```python
from build123d import *

# Parameters (mm, degrees)
F0_W     = 457.2
F0_H     = 304.8
F0_R     = 6.35
F1_DEPTH = 6.35
F2_W     = 2.54
F2_H     = 5.08
F3_DEPTH = 2.54


with BuildPart() as f1:
    # F0 (on Top) → F1 (new body)
    with BuildSketch(Plane.XY):
        with Locations((228.6, -152.4)):
            Rectangle(F0_W, F0_H)
        with Locations((25.4, -272.70785)):
            Circle(F0_R, mode=Mode.SUBTRACT)
        with Locations((76.2, -272.70785)):
            Circle(F0_R, mode=Mode.SUBTRACT)
        with Locations((127, -272.70785)):
            Circle(F0_R, mode=Mode.SUBTRACT)
        with Locations((177.8, -272.70785)):
            Circle(F0_R, mode=Mode.SUBTRACT)
        with Locations((25.4, -221.90785)):
            Circle(F0_R, mode=Mode.SUBTRACT)
        with Locations((76.2, -221.90785)):
            Circle(F0_R, mode=Mode.SUBTRACT)
        with Locations((25.4, -171.10785)):
            Circle(F0_R, mode=Mode.SUBTRACT)
        with Locations((76.2, -171.10785)):
            Circle(F0_R, mode=Mode.SUBTRACT)
        with Locations((127, -221.90785)):
            Circle(F0_R, mode=Mode.SUBTRACT)
        with Locations((177.8, -221.90785)):
            Circle(F0_R, mode=Mode.SUBTRACT)
        with Locations((127, -171.10785)):
            Circle(F0_R, mode=Mode.SUBTRACT)
        with Locations((177.8, -171.10785)):
            Circle(F0_R, mode=Mode.SUBTRACT)
        with Locations((228.6, -272.70785)):
            Circle(F0_R, mode=Mode.SUBTRACT)
        with Locations((279.4, -272.70785)):
            Circle(F0_R, mode=Mode.SUBTRACT)
        with Locations((330.2, -272.70785)):
            Circle(F0_R, mode=Mode.SUBTRACT)
        with Locations((381, -272.70785)):
            Circle(F0_R, mode=Mode.SUBTRACT)
        with BuildLine():
            ThreePointArc((438.15, -272.70785), (427.309872, -277.197978), (431.8, -266.35785))
            Line((431.8, -266.35785), (431.8, -262.54785))
            Line((431.8, -262.54785), (444.5, -262.54785))
            Line((444.5, -262.54785), (444.5, -272.70785))
            Line((444.5, -272.70785), (438.15, -272.70785))
        make_face(mode=Mode.SUBTRACT)
        with Locations((228.6, -221.90785)):
            Circle(F0_R, mode=Mode.SUBTRACT)
        with Locations((279.4, -221.90785)):
            Circle(F0_R, mode=Mode.SUBTRACT)
        with Locations((330.2, -221.90785)):
            Circle(F0_R, mode=Mode.SUBTRACT)
        with Locations((228.6, -171.10785)):
            Circle(F0_R, mode=Mode.SUBTRACT)
        with Locations((279.4, -171.10785)):
            Circle(F0_R, mode=Mode.SUBTRACT)
        with Locations((330.2, -171.10785)):
            Circle(F0_R, mode=Mode.SUBTRACT)
        with Locations((381, -221.90785)):
            Circle(F0_R, mode=Mode.SUBTRACT)
        with Locations((431.8, -221.90785)):
            Circle(F0_R, mode=Mode.SUBTRACT)
        with Locations((381, -171.10785)):
            Circle(F0_R, mode=Mode.SUBTRACT)
        with Locations((431.8, -171.10785)):
            Circle(F0_R, mode=Mode.SUBTRACT)
        with Locations((25.4, -120.30785)):
            Circle(F0_R, mode=Mode.SUBTRACT)
        with Locations((76.2, -120.30785)):
            Circle(F0_R, mode=Mode.SUBTRACT)
        with Locations((127, -120.30785)):
            Circle(F0_R, mode=Mode.SUBTRACT)
        with Locations((177.8, -120.30785)):
            Circle(F0_R, mode=Mode.SUBTRACT)
        with Locations((25.4, -69.50785)):
            Circle(F0_R, mode=Mode.SUBTRACT)
        with Locations((76.2, -69.50785)):
            Circle(F0_R, mode=Mode.SUBTRACT)
        with Locations((25.4, -18.70785)):
            Circle(F0_R, mode=Mode.SUBTRACT)
        with Locations((76.2, -18.70785)):
            Circle(F0_R, mode=Mode.SUBTRACT)
        with Locations((127, -69.50785)):
            Circle(F0_R, mode=Mode.SUBTRACT)
        with Locations((177.8, -69.50785)):
            Circle(F0_R, mode=Mode.SUBTRACT)
        with Locations((127, -18.70785)):
            Circle(F0_R, mode=Mode.SUBTRACT)
        with Locations((177.8, -18.70785)):
            Circle(F0_R, mode=Mode.SUBTRACT)
        with Locations((228.6, -120.30785)):
            Circle(F0_R, mode=Mode.SUBTRACT)
        with Locations((279.4, -120.30785)):
            Circle(F0_R, mode=Mode.SUBTRACT)
        with Locations((330.2, -120.30785)):
            Circle(F0_R, mode=Mode.SUBTRACT)
        with Locations((381, -120.30785)):
            Circle(F0_R, mode=Mode.SUBTRACT)
        with Locations((431.8, -120.30785)):
            Circle(F0_R, mode=Mode.SUBTRACT)
        with Locations((228.6, -69.50785)):
            Circle(F0_R, mode=Mode.SUBTRACT)
        with Locations((279.4, -69.50785)):
            Circle(F0_R, mode=Mode.SUBTRACT)
        with Locations((330.2, -69.50785)):
            Circle(F0_R, mode=Mode.SUBTRACT)
        with Locations((228.6, -18.70785)):
            Circle(F0_R, mode=Mode.SUBTRACT)
        with Locations((279.4, -18.70785)):
            Circle(F0_R, mode=Mode.SUBTRACT)
        with Locations((330.2, -18.70785)):
            Circle(F0_R, mode=Mode.SUBTRACT)
        with Locations((381, -69.50785)):
            Circle(F0_R, mode=Mode.SUBTRACT)
        with Locations((431.8, -69.50785)):
            Circle(F0_R, mode=Mode.SUBTRACT)
        with Locations((381, -18.70785)):
            Circle(F0_R, mode=Mode.SUBTRACT)
        with BuildLine():
            ThreePointArc((431.8, -25.05785), (427.309872, -14.217722), (438.15, -18.70785))
            Line((438.15, -18.70785), (444.5, -18.70785))
            Line((444.5, -18.70785), (444.5, -28.86785))
            Line((444.5, -28.86785), (431.8, -28.86785))
            Line((431.8, -28.86785), (431.8, -25.05785))
        make_face(mode=Mode.SUBTRACT)
    extrude(amount=F1_DEPTH)

    # F2 (on face) → F3 (cut)
    with BuildSketch(Plane.YZ.offset(457.2)):
        with Locations((-151.13, 2.54)):
            Rectangle(F2_W, F2_H)
    extrude(amount=-F3_DEPTH, mode=Mode.SUBTRACT)


solid = f1.part
```
Can you work these out from the model? Positions are in its coordinate system, mm. Coordinates: 2 decimals unless noted, no trailing zeros. Order: outer loops, then holes, each group sorted by start corner. A loop starts at its lowest first (then second) coordinate and runs counter-clockwise, first axis right, second up. Notation, with made-up numbers: (-1, 7.5) -> (18, 7.5) arc R13 cw to (18, 12.5) -> close; hole circle Ø1 at (-12, 72). An arc over 180 degrees is marked (long way). Write each question's results on one line, items separated by ' | '.
Item 1: I want a section at B-B, the plane z = 2.25. Count the separate pieces of the cut face and the enclosed holes in it, then the cut area to 3 significant figures.
Results are:
separate pieces: 1 | enclosed holes: 54 | area: 132,000 mm²
Item 2: I'm going to push a flat-ended pin straight in: pin 1 Ø6 at (x, y) = (299, -269.5) entering from -Z. Where does the tip first touch, or does it pass through?
Results are:
pin 1: z = 0
Item 3: I want a section at A-A, the plane x = 76.2. Write out the boundary of the cut face in (y, z).
Results are:
outline: (-304.8, 0) -> (-279.06, 0) -> (-279.06, 6.35) -> (-304.8, 6.35) -> close; (-266.36, 0) -> (-228.26, 0) -> (-228.26, 6.35) -> (-266.36, 6.35) -> close; (-215.56, 0) -> (-177.46, 0) -> (-177.46, 6.35) -> (-215.56, 6.35) -> close; (-164.76, 0) -> (-126.66, 0) -> (-126.66, 6.35) -> (-164.76, 6.35) -> close; (-113.96, 0) -> (-75.86, 0) -> (-75.86, 6.35) -> (-113.96, 6.35) -> close; (-63.16, 0) -> (-25.06, 0) -> (-25.06, 6.35) -> (-63.16, 6.35) -> close; (-12.36, 0) -> (0, 0) -> (0, 6.35) -> (-12.36, 6.35) -> close
